```python
from build123d import *

# Parameters (mm, degrees)
BOSS_EXTRU_1_DEPTH      = 1.6
CONG_1_R                = 2
EXTRU_MINCE1_DEPTH      = 1.6
EXTRU_MINCE1_DEPTH_BACK = 20


with BuildPart() as part:
    # Balayage1: sweep along a path in Esquisse1
    with BuildLine(Plane.XY) as balayage1_path:
        Line((-26, 27), (26, 27))
        ThreePointArc((26, 27), (33.071067812, 24.071067812), (36, 17))
        Line((36, 17), (36, -17))
        ThreePointArc((36, -17), (33.071067812, -24.071067812), (26, -27))
        Line((26, -27), (-26, -27))
        ThreePointArc((-26, -27), (-33.071067812, -24.071067812), (-36, -17))
        Line((-36, -17), (-36, 17))
        ThreePointArc((-36, 17), (-33.071067812, 24.071067812), (-26, 27))
    # profil → Balayage1 (sweep)
    with BuildSketch(Plane(origin=(0, 0, 0), x_dir=(0, 0, -1), z_dir=(1, 0, 0))):
        Polygon((0, -25.521907401), (4.110600662, -25.521907401), (10, -21), (10, -21.4), (9.8, -21.4), (9.8, -22.2), (10, -22.2), (10, -22.6), (10.4, -22.6), (10.4, -23), (10.8, -23), (10.8, -23.4), (11.2, -23.4), (11.2, -23.8), (11.6, -23.8), (11.6, -24.2), (11.2, -24.2), (11.2, -24.6), (10.8, -24.6), (10.8, -25), (10.4, -25), (10.4, -25.4), (10, -25.4), (10, -25.8), (9.8, -25.8), (9.8, -26.6), (10, -26.6), (10, -27), (0, -27), align=None)
    sweep(path=balayage1_path.line)

    # Esquisse1<3> → Boss.-Extru.1 (add)
    with BuildSketch(Plane.XY):
        with BuildLine():
            Line((-26, 27), (26, 27))
            ThreePointArc((26, 27), (33.071067812, 24.071067812), (36, 17))
            Line((36, 17), (36, -17))
            ThreePointArc((36, -17), (33.071067812, -24.071067812), (26, -27))
            Line((26, -27), (-26, -27))
            ThreePointArc((-26, -27), (-33.071067812, -24.071067812), (-36, -17))
            Line((-36, -17), (-36, 17))
            ThreePointArc((-36, 17), (-33.071067812, 24.071067812), (-26, 27))
        make_face()
    extrude(amount=BOSS_EXTRU_1_DEPTH)

    # Congé1
    cong_1_edges = [part.edges().sort_by_distance(p)[0] for p in [
        (34.521907401, 0, 0),
        (32.025898512, -23.025898512, 0),
        (0, -25.521907401, 0),
        (-32.025898512, -23.025898512, 0),
        (-34.521907401, 0, 0),
        (-32.025898512, 23.025898512, 0),
        (0, 25.521907401, 0),
        (0, -25.521907401, 0),
        (32.025898512, 23.025898512, 0),
    ]]
    fillet(cong_1_edges, radius=CONG_1_R)

    # Esquisse2 → Extru.-Mince1 (add, two sides)
    with BuildSketch(Plane.XY) as extru_mince1_sk:
        with BuildLine():
            Line((-36.4, 17), (-36.4, -17))
            ThreePointArc((-36.4, -17), (-33.353910524, -24.353910524), (-26, -27.4))
            Line((-26, -27.4), (26, -27.4))
            ThreePointArc((26, -27.4), (33.353910524, -24.353910524), (36.4, -17))
            Line((36.4, -17), (36.4, 17))
            ThreePointArc((36.4, 17), (33.353910524, 24.353910524), (26, 27.4))
            Line((26, 27.4), (-26, 27.4))
            ThreePointArc((-26, 27.4), (-33.353910524, 24.353910524), (-36.4, 17))
        make_face()
        with BuildLine():
            Line((-36, 17), (-36, -17))
            ThreePointArc((-36, -17), (-33.071067812, -24.071067812), (-26, -27))
            Line((-26, -27), (26, -27))
            ThreePointArc((26, -27), (33.071067812, -24.071067812), (36, -17))
            Line((36, -17), (36, 17))
            ThreePointArc((36, 17), (33.071067812, 24.071067812), (26, 27))
            Line((26, 27), (-26, 27))
            ThreePointArc((-26, 27), (-33.071067812, 24.071067812), (-36, 17))
        make_face(mode=Mode.SUBTRACT)
    extrude(amount=EXTRU_MINCE1_DEPTH)
    extrude(extru_mince1_sk.sketch, amount=-EXTRU_MINCE1_DEPTH_BACK)


solid = part.part
```
Part model, mm, in its own coordinate system. A direction names the side the tool comes from. Give positions to 0.01 mm unless a question says otherwise; leave off trailing zeros. Write each loop counter-clockwise with the first axis right and the second up, starting at its lowest first coordinate (ties: lowest second). Pieces come first, ordered by that corner, then holes. Notation, with made-up numbers: (68, 88) -> (105, 88) arc R28 cw to (105, 114) -> close; hole circle Ø7 at (-23.75, 79.25). An arc over 180 degrees is marked (long way). Put each result on its own line as item: value. Start each with the question number.
Item 1: Pin check, flat tips, straight feed: pin 1 Ø6 at (x, y) = (7.5, 14) entering from -Z; pin 2 Ø10 at (y, z) = (-20.5, -11) entering from +X. Stop position of each tip, or through.
Item 2: Cut at A-A (z = -18). List the corners of the cut face in (x, y), then the cut area to 3 significant figures.
Item 3: Pull direction X, two halves, no side cores. Call faces 4 (the face through (36.4, 0, -9)), 5 (the face through (0, -27.4, -9)), 6 (the face through (30.48, 21.57, -11)): pulls with the +X half, pulls with the -X half, needs draft (parallel to the pull), parting line crosses it, or undercut.
Item 4: Which spindle directions (+Z, -Z, +X, -X, +Y, -Y) get a long thin tool onto all of the face, cutting with end or side? Do faces 1 (the face through (33.273, -24.434, -9.049)), 2 (the face through (32.229, -0.238, -7.097)), 3 (the face through (30.289, -21.196, -10.597)). Say none if no direction does.
Item 5: Wall check: L1, parallel to X at y = -13.5, z = -11; L2, parallel to X at y = -11.5, z = -15; L3, parallel to Y at x = -12, z = -15.25. Give the ranges that are in metal, low to high. Write a range as [from, to].
Item 6: Cut at B-B (z = -8.5). List the corners of the cut face in (x, y).
Answer list:
1. pin 1: stops at z = 0
1. pin 2: stops at x = 36.4
2. outline: (-36.4, -17) arc R10.4 ccw to (-26, -27.4) -> (26, -27.4) arc R10.4 ccw to (36.4, -17) -> (36.4, 17) arc R10.4 ccw to (26, 27.4) -> (-26, 27.4) arc R10.4 ccw to (-36.4, 17) -> close; hole (-36, -17) arc R10 ccw to (-26, -27) -> (26, -27) arc R10 ccw to (36, -17) -> (36, 17) arc R10 ccw to (26, 27) -> (-26, 27) arc R10 ccw to (-36, 17) -> close
2. area: 94.4 mm2
3. face 4: pulls with the +X half
3. face 5: needs draft
3. face 6: undercut
4. face 1: +Z, -Z, +X, -Y
4. face 2: none
4. face 3: -Z
5. L1: x = [-36.4, -36], [-33.6, -32.4], [32.4, 33.6], [36, 36.4]
5. L2: x = [-36.4, -36], [36, 36.4]
5. L3: y = [-27.4, -27], [27, 27.4]
6. outline: (-36.4, -17) arc R10.4 ccw to (-26, -27.4) -> (26, -27.4) arc R10.4 ccw to (36.4, -17) -> (36.4, 17) arc R10.4 ccw to (26, 27.4) -> (-26, 27.4) arc R10.4 ccw to (-36.4, 17) -> close; hole (-31.15, -17) arc R5.15 ccw to (-26, -22.15) -> (26, -22.15) arc R5.15 ccw to (31.15, -17) -> (31.15, 17) arc R5.15 ccw to (26, 22.15) -> (-26, 22.15) arc R5.15 ccw to (-31.15, 17) -> close
